Verification items for the finished model (mm, model axes). Face numbers are marked on the shaded views. A direction names the side the tool comes from. Round coordinates to 2 decimals unless told otherwise and drop trailing zeros. Write each loop counter-clockwise with the first axis right and the second up, starting at its lowest first coordinate (ties: lowest second). Pieces come first, ordered by that corner, then holes. Notation, with made-up numbers: (-4, -36) - (54, -36) arc R7 ccw to (54, -32) - close; hole circle Ø6 at (40, 65.5). An arc over 180 degrees is marked (long way). Answer as a JSON object with one key per item and string values. Group by question number.
1) Section check D-D (x = 14.5). Enter the section's corners in (y, z), then the cut area to 3 significant figures.
2) Section check A-A (x = 53.5). Enter the section's corners in (y, z), then the cut area to 3 significant figures.
3) Section check C-C (y = 17.5). Enter the section's corners in (x, z).
4) Section check B-B (y = -2). Enter the section's corners in (x, z).
5) Go/stop test with flat-tipped pins: pin 1 Ø1.5 at (y, z) = (2, 4) entering from +X; pin 2 Ø3 at (x, z) = (45.5, 3) entering from -Y; pin 3 Ø0.8 at (y, z) = (47, 2) entering from -X. Record where each tip stops, or that it passes through.
6) Thickness scan on line 1 (Y direction, x = 53, z = 3.75); line 2 (Y direction, x = 37, z = 4.75); line 3 (X direction, y = 0.5, z = 1). Record the ranges inside material, lowest first.
7) Set-up check for the marked faces 1 and 2: record each of +Z, -Z, +X, -X, +Y, -Y from which the full face is reachable in a straight line by a thin tool's end or side.
Autodesk Inventor part; units mm, degrees
ref_plane "YZ Plane" through (0, 0, 0) normal (1, 0, 0) x (0, 1, 0)
ref_plane "XZ Plane" through (0, 0, 0) normal (0, 1, 0) x (-1, 0, 0)
ref_plane "XY Plane" through (0, 0, 0) normal (0, 0, 1) x (1, 0, 0)
sketch "Sketch1" plane through (0, 0, 0) normal (0, 0, 1) x (1, 0, 0)
  line L0 (0, 0) -> (52, 0)
  line L1 (52, 0) -> (52, 69)
  line L2 (52, 69) -> (34, 69)
  line L3 (34, 69) -> (0, 6)
  line L4 (0, 6) -> (0, 0)
  dimension "d0" = 52
  dimension "d1" = 6
  dimension "d2" = 18
  dimension "d3" = 69
extrude "Extrusion1" add sketch "Sketch1" along normal blind 6.5
sketch "Sketch2" plane through (0, 0, 6.5) normal (0, 0, 1) x (1, 0, 0)
  line L0 (0, 0) -> (52, 0)
  line L1 (52, 0) -> (52, 69)
  line L2 (18.75, 16.3) -> (23.25, 16.3)
  line L3 (23.25, 0) -> (18.75, 0)
  line L4 (25.75, 12.3) -> (25.75, 5)
  line L5 (16.25, 5) -> (16.25, 12.3)
  line L6 (39.7, 55.25) -> (47, 55.25)
  line L7 (47, 45.75) -> (39.7, 45.75)
  line L8 (52, 52.75) -> (52, 48.25)
  line L9 (35.7, 48.25) -> (35.7, 52.75)
  line L10 (16.25, 12.3) -> (18.75, 12.3)
  line L11 (23.25, 12.3) -> (25.75, 12.3)
  line L12 (18.75, 0) -> (18.75, 5)
  line L13 (18.75, 12.3) -> (18.75, 16.3)
  line L14 (25.75, 5) -> (23.25, 5)
  line L15 (18.75, 5) -> (16.25, 5)
  line L16 (23.25, 16.3) -> (23.25, 12.3)
  line L17 (23.25, 5) -> (23.25, 0)
  line L18 (52, 48.25) -> (47, 48.25)
  line L19 (39.7, 48.25) -> (35.7, 48.25)
  line L20 (35.7, 52.75) -> (39.7, 52.75)
  line L21 (47, 52.75) -> (52, 52.75)
  line L22 (39.7, 45.75) -> (39.7, 48.25)
  line L23 (39.7, 52.75) -> (39.7, 55.25)
  line L24 (47, 55.25) -> (47, 52.75)
  line L25 (47, 48.25) -> (47, 45.75)
  point P0 (35.7, 50.5)
  point P1 (21, 16.3)
  dimension "d6" = 4.5
  dimension "d7" = 2.5
  dimension "d8" = 2.5
  dimension "d9" = 5
  dimension "d10" = 4
  dimension "d11" = 7.3
  dimension "d12" = 4.5
  dimension "d13" = 2.5
  dimension "d14" = 2.5
  dimension "d15" = 4
  dimension "d16" = 5
  dimension "d17" = 7.3
  dimension "d19" = 31
  dimension "d39" = 18.5
extrude "Extrusion2" cut sketch "Sketch2" against normal blind 6.5
sketch "Sketch3" plane through (0, 0, 6.5) normal (0, 0, 1) x (1, 0, 0)
  line L0 (23.25, 0) -> (52, 0)
  line L1 (52, 0) -> (52, 48.25)
  line L2 (35.7, 48.25) -> (35.7, 52.75)
  line L3 (52, 52.75) -> (52, 69)
  line L4 (0, 0) -> (18.75, 0)
  line L5 (18.75, 16.3) -> (23.25, 16.3)
  line L6 (5.5, 0) -> (13.5, 0)
  line L7 (13.5, 0) -> (13.5, -4.5)
  line L8 (11.5, -6.5) -> (7.5, -6.5)
  line L9 (5.5, -4.5) -> (5.5, 0)
  line L10 (28.5, 0) -> (36.5, 0)
  line L11 (36.5, 0) -> (36.5, -4.5)
  line L12 (34.5, -6.5) -> (30.5, -6.5)
  line L13 (28.5, -4.5) -> (28.5, 0)
  line L14 (52, 35) -> (56.5, 35)
  line L15 (58.5, 37) -> (58.5, 41)
  line L16 (56.5, 43) -> (52, 43)
  line L17 (52, 43) -> (52, 35)
  line L18 (52, 66) -> (56.5, 66)
  line L19 (58.5, 64) -> (58.5, 60)
  line L20 (56.5, 58) -> (52, 58)
  line L21 (52, 58) -> (52, 66)
  arc A0 (5.5, -4.5) -> (7.5, -6.5) centre (7.5, -4.5) ccw
  arc A1 (11.5, -6.5) -> (13.5, -4.5) centre (11.5, -4.5) ccw
  arc A2 (28.5, -4.5) -> (30.5, -6.5) centre (30.5, -4.5) ccw
  arc A3 (34.5, -6.5) -> (36.5, -4.5) centre (34.5, -4.5) ccw
  arc A4 (56.5, 35) -> (58.5, 37) centre (56.5, 37) ccw
  arc A5 (58.5, 41) -> (56.5, 43) centre (56.5, 41) ccw
  arc A6 (58.5, 64) -> (56.5, 66) centre (56.5, 64) ccw
  arc A7 (56.5, 58) -> (58.5, 60) centre (56.5, 60) ccw
  point P0 (35.7, 50.5)
  point P1 (21, 16.3)
  dimension "d22" = 2
  dimension "d23" = 6.5
  dimension "d24" = 8
  dimension "d25" = 8
  dimension "d26" = 8
  dimension "d27" = 8
  dimension "d28" = 6.5
  dimension "d29" = 7.5
  dimension "d30" = 15
  dimension "d31" = 15
  dimension "d32" = 7.5
extrude "Extrusion3" add sketch "Sketch3" against normal blind 6.5
sketch "Sketch4" plane through (0, 0, 6.5) normal (0, 0, 1) x (1, 0, 0)
  line L0 (52, 0) -> (40, 0)
  line L1 (40, 0) -> (40, 12)
  line L2 (40, 12) -> (52, 12)
  line L3 (52, 12) -> (52, 0)
  dimension "d35" = 12
  dimension "d36" = 12
extrude "Extrusion4" cut sketch "Sketch4" against normal blind 6.5
chamfer "Chamfer1" distance 2 angle 45 1 edges at (40, 12, 3.25)
properties part number "x_motor_cable_mount_brace" material "Plywood, Finish"
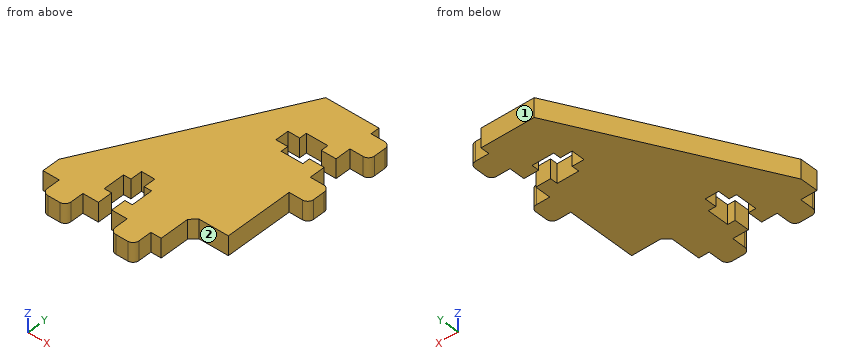
Returned:
{
 "1": {"outline": "(0, 0) - (32.87, 0) - (32.87, 6.5) - (0, 6.5) - close", "area": "214 mm2"},
 "2": {"outline": "(35, 0) - (43, 0) - (43, 6.5) - (35, 6.5) - close; (58, 0) - (66, 0) - (66, 6.5) - (58, 6.5) - close", "area": "104 mm2"},
 "3": {"outline": "(6.21, 0) - (52, 0) - (52, 6.5) - (6.21, 6.5) - close"},
 "4": {"outline": "(5.5, 0) - (13.5, 0) - (13.5, 6.5) - (5.5, 6.5) - close; (28.5, 0) - (36.5, 0) - (36.5, 6.5) - (28.5, 6.5) - close"},
 "5": {"pin 1": "x = 40", "pin 2": "y = 12", "pin 3": "x = 21.91"},
 "6": {"line 1": "35 to 43, 58 to 66", "line 2": "0 to 48.25, 52.75 to 69", "line 3": "0 to 18.75, 23.25 to 40"},
 "7": {"face 1": "+Z, -Z, +X, -X, +Y", "face 2": "+Z, -Z, +X, -Y"}
}
